Input: part model. Units: mm. Frame: model coordinates. Face numbers are marked on the shaded views. A direction names the side the tool comes from. Round coordinates to 2 decimals unless told otherwise and drop trailing zeros. Order: outer loops, then holes, each group sorted by start corner. A loop starts at its lowest first (then second) coordinate and runs counter-clockwise, first axis right, second up. Notation, with made-up numbers: (88, 28) -> (133, 28) arc R10 ccw to (133, 33) -> close; hole circle Ø8 at (-22.75, 29). An arc over 180 degrees is marked (long way). Use a Markdown table: item, result.
from build123d import *

# Parameters (mm, degrees)
BOSS_EXTRUDE1_DEPTH = 18.8
CUT_EXTRUDE2_DEPTH  = 11.9
BOSS_EXTRUDE2_DEPTH = 6.4
SKETCH9_R           = 1.2075
CUT_EXTRUDE3_DEPTH  = 2.5
SKETCH9_4_R         = 3.05
SKETCH9_4_R_2       = 1.2075
BOSS_EXTRUDE5_DEPTH = 4
SKETCH11_R          = 2.25
CUT_EXTRUDE8_DEPTH  = 3.6
BOSS_EXTRUDE6_DEPTH = 4.5
CUT_EXTRUDE9_DEPTH  = 11.9
CUT_EXTRUDE10_DEPTH = 11.9


with BuildPart() as part:
    # Sketch2 → Boss-Extrude1 (new body)
    with BuildSketch(Plane(origin=(0, 0, 0), x_dir=(1, 0, 0), z_dir=(0, 1, 0))):
        with BuildLine():
            ThreePointArc((-5.105212739, -6.0942024), (5.62149891, 5.62149891), (-6.0942024, -5.105212739))
            ThreePointArc((-6.0942024, -5.105212739), (-6.116473657, -6.116473657), (-5.105212739, -6.0942024))
        make_face()
        with BuildLine():
            Line((-3.42, 1.6), (3.42, 1.6))
            ThreePointArc((3.42, 1.6), (4.339238816, 1.219238816), (4.72, 0.3))
            Line((4.72, 0.3), (4.72, -0.3))
            ThreePointArc((4.72, -0.3), (4.339238816, -1.219238816), (3.42, -1.6))
            Line((3.42, -1.6), (-3.42, -1.6))
            ThreePointArc((-3.42, -1.6), (-4.339238816, -1.219238816), (-4.72, -0.3))
            Line((-4.72, -0.3), (-4.72, 0.3))
            ThreePointArc((-4.72, 0.3), (-4.339238816, 1.219238816), (-3.42, 1.6))
        make_face(mode=Mode.SUBTRACT)
    extrude(amount=BOSS_EXTRUDE1_DEPTH)

    # Sketch3 → Cut-Extrude2 (cut)
    with BuildSketch(Plane(origin=(0, 0, 0), x_dir=(1, 0, 0), z_dir=(0, 1, 0))):
        with BuildLine():
            Line((-5.98, 3.733912158), (-5.98, -3.733912158))
            ThreePointArc((-5.98, -3.733912158), (-4.924640659, -5.044840372), (-3.588648771, -6.068286414))
            ThreePointArc((-3.588648771, -6.068286414), (3.493030644, -6.12382535), (7.05, 0))
            ThreePointArc((7.05, 0), (1.94209938, 6.777222883), (-5.98, 3.733912158))
        make_face()
        with BuildLine():
            Line((-4.72, -0.3), (-4.72, 0.3))
            ThreePointArc((-4.72, 0.3), (-4.339238816, 1.219238816), (-3.42, 1.6))
            Line((-3.42, 1.6), (3.42, 1.6))
            ThreePointArc((3.42, 1.6), (4.339238816, 1.219238816), (4.72, 0.3))
            Line((4.72, 0.3), (4.72, -0.3))
            ThreePointArc((4.72, -0.3), (4.339238816, -1.219238816), (3.42, -1.6))
            Line((3.42, -1.6), (-3.42, -1.6))
            ThreePointArc((-3.42, -1.6), (-4.339238816, -1.219238816), (-4.72, -0.3))
        make_face(mode=Mode.SUBTRACT)
    extrude(amount=CUT_EXTRUDE2_DEPTH, mode=Mode.SUBTRACT)

    # Sketch4 → Boss-Extrude2 (add)
    with BuildSketch(Plane.XZ):
        with BuildLine():
            Line((-2.25, 6.681317235), (-2.25, 2.85))
            Line((-2.25, 2.85), (2.25, 2.85))
            Line((2.25, 2.85), (2.25, 6.681317235))
            ThreePointArc((2.25, 6.681317235), (0, 7.05), (-2.25, 6.681317235))
        make_face()
    extrude(amount=-BOSS_EXTRUDE2_DEPTH)

    # Sketch9 → Cut-Extrude3 (cut)
    with BuildSketch(Plane(origin=(0, 0, 2.85), x_dir=(-1, 0, 0), z_dir=(0, 0, -1))):
        with Locations((0, 3.2)):
            Circle(SKETCH9_R)
    extrude(amount=-CUT_EXTRUDE3_DEPTH, mode=Mode.SUBTRACT)

    # Sketch9_4 → Boss-Extrude5 (add)
    with BuildSketch(Plane(origin=(0, 0, 2.85), x_dir=(-1, 0, 0), z_dir=(0, 0, -1))):
        with Locations((0, 3.2)):
            Circle(SKETCH9_4_R)
        with Locations((0, 3.2)):
            Circle(SKETCH9_4_R_2, mode=Mode.SUBTRACT)
    extrude(amount=-BOSS_EXTRUDE5_DEPTH)

    # Sketch11 → Cut-Extrude8 (cut, through all)
    with BuildSketch(Plane(origin=(0, 0, 5.35), x_dir=(-1, 0, 0), z_dir=(0, 0, -1))):
        with Locations((0, 3.25)):
            Circle(SKETCH11_R)
    extrude(amount=-CUT_EXTRUDE8_DEPTH, mode=Mode.SUBTRACT)

    # Sketch15 → Boss-Extrude6 (add)
    with BuildSketch(Plane.ZY.offset(2.25)):
        Polygon((2.85, 6.4), (7.35, 6.4), (7.35, 10.9), align=None)
    extrude(amount=-BOSS_EXTRUDE6_DEPTH)

    # Sketch3_3 → Cut-Extrude9 (cut)
    with BuildSketch(Plane(origin=(0, 0, 0), x_dir=(1, 0, 0), z_dir=(0, 1, 0))):
        with BuildLine():
            ThreePointArc((-5.98, 3.733912158), (-7.05, 0), (-5.98, -3.733912158))
            Line((-5.98, -3.733912158), (-5.98, 3.733912158))
        make_face()
    extrude(amount=CUT_EXTRUDE9_DEPTH, mode=Mode.SUBTRACT)

    # Sketch16 → Cut-Extrude10 (cut)
    with BuildSketch(Plane.XZ):
        Polygon((7.95, -7.95), (-7.95, -7.95), (-7.95, 0), (-7.95, 1.6), (7.95, 1.6), (7.95, 0), align=None)
    extrude(amount=-CUT_EXTRUDE10_DEPTH, mode=Mode.SUBTRACT)


solid = part.part
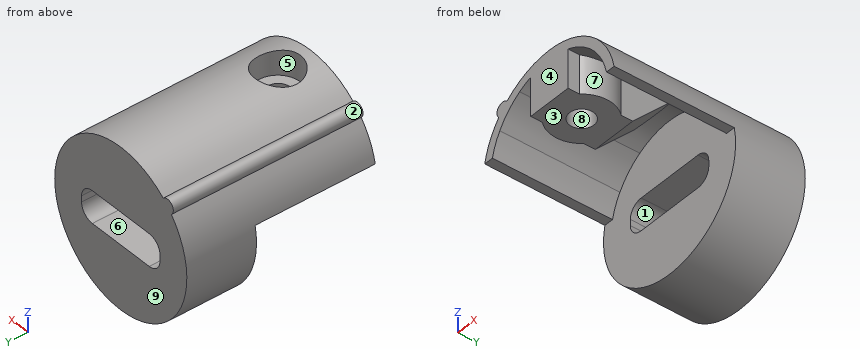
1) Ray query, probe 1 along Z at (x, y) = (-0.25, 15); probe 2 along Y at (x, z) = (0, 7.4); probe 3 along Y at (x, z) = (0, 4.25). Return the intervals inside material, ascending.
Answer key:
| item | result |
|---|---|
| probe 1 | z = -7.95 to -1.6, 1.6 to 7.95 |
| probe 2 | y = 0 to 1, 5.5 to 18.8 |
| probe 3 | y = 0 to 1.99, 4.41 to 7.8, 11.9 to 18.8 |
2) Contact query for flat-ended pins moving along their axis: P1, Ø6, axis at y = 15.5, z = 2.5, coming from the -X side; P2, Ø3, axis at x = -0.5, y = 4.5, coming from the -Z side; P3, Ø2.5, axis at x = 0, y = 3.25, coming from the +Z side; P4, Ø1.5, axis at x = -3, y = 15, coming from the +Z side. Output: stop coordinate, or through.
Answer key:
| item | result |
|---|---|
| P1 | stops at x = -7.95 |
| P2 | stops at z = 2.85 |
| P3 | stops at z = 5.35 |
| P4 | stops at z = 7.62 |
3) Cut plane B-B on z = 0. Return loops of the section in (x, y), and give its area (3 significant figures).
Answer key:
| item | result |
|---|---|
| outline | (-7.95, 11.9) -> (-4.72, 11.9) -> (-4.72, 18.8) -> (-7.95, 18.8) -> close; (4.72, 11.9) -> (7.95, 11.9) -> (7.95, 18.8) -> (4.72, 18.8) -> close |
| area | 44.6 mm^2 |
4) Cut plane A-A on x = 0. Return loops of the section in (y, z).
Answer key:
| item | result |
|---|---|
| outline | (0, 2.85) -> (1.99, 2.85) -> (1.99, 5.35) -> (1, 5.35) -> (1, 7.95) -> (0, 7.95) -> close; (4.41, 2.85) -> (6.4, 2.85) -> (10.6, 7.05) -> (11.9, 7.05) -> (11.9, 1.6) -> (18.8, 1.6) -> (18.8, 7.95) -> (5.5, 7.95) -> (5.5, 5.35) -> (4.41, 5.35) -> close; (11.9, -7.95) -> (18.8, -7.95) -> (18.8, -1.6) -> (11.9, -1.6) -> close |
5) Draft query along Z for the marked faces 1, 2, 3 and 4. Return one class per face: released by +Z, released by -Z, zero draft, split by the parting line, or undercut.
Answer key:
| item | result |
|---|---|
| face 1 | undercut |
| face 2 | undercut |
| face 3 | released by -Z |
| face 4 | zero draft |
6) Set-up query: the marked faces 5, 6, 7, 8 and 9. Return all of +Z, -Z, +X, -X, +Y, -Y with unobstructed straight access to the full face (end or side cutting, diameter ignored); none if empty.
Answer key:
| item | result |
|---|---|
| face 5 | +Z |
| face 6 | +Y, -Y |
| face 7 | -Z |
| face 8 | +Z, -Z |
| face 9 | +Z, -Z, +X, -X, +Y |
7) Cut plane C-C on y = 12.25. Return loops of the section in (x, z), and give its area (3 significant figures).
Answer key:
| item | result |
|---|---|
| outline | (-6.09, 5.11) arc R7.95 ccw (long way) to (-5.11, 6.09) arc R0.7 ccw (long way) to start; hole (-4.72, -0.3) arc R1.3 ccw to (-3.42, -1.6) -> (3.42, -1.6) arc R1.3 ccw to (4.72, -0.3) -> (4.72, 0.3) arc R1.3 ccw to (3.42, 1.6) -> (-3.42, 1.6) arc R1.3 ccw to (-4.72, 0.3) -> close |
| area | 171 mm^2 |
8) Cut plane D-D on x = 2.5. Return loops of the section in (y, z), and give its area (3 significant figures).
Answer key:
| item | result |
|---|---|
| outline | (0, 6.59) -> (1.45, 6.59) -> (1.45, 2.85) -> (4.95, 2.85) -> (4.95, 6.59) -> (11.9, 6.59) -> (11.9, 1.6) -> (18.8, 1.6) -> (18.8, 7.55) -> (0, 7.55) -> close; (11.9, -7.55) -> (18.8, -7.55) -> (18.8, -1.6) -> (11.9, -1.6) -> close |
| area | 107 mm^2 |
